Part model, mm, in its own coordinate system. Face numbers are marked on the shaded views. A direction names the side the tool comes from. Give positions to 0.01 mm unless a question says otherwise; leave off trailing zeros. Write each loop counter-clockwise with the first axis right and the second up, starting at its lowest first coordinate (ties: lowest second). Pieces come first, ordered by that corner, then holes. Notation, with made-up numbers: M 17,-27.75 L 24,-27.75 A24 cw 24,2.25 Z; hole C 51,-21.75 d9. An arc over 180 degrees is marked long. Answer as CSV lines item,"result". Start each with the question number.
Item 1: Band-saw the part on C-C, the plane x = -18.5. List the corners of the cut face in (y, z).
Item 2: 3-axis set-ups, long thin cutter, end or side, ignore diameter. For the marked faces 4 and 5: which of +Z, -Z, +X, -X, +Y, -Y reach the whole face in a straight line?
Item 3: Band-saw the part on A-A, the plane z = 10. List the corners of the cut face in (x, y), then the cut area to 3 significant figures.
Item 4: Band-saw the part on B-B, the plane x = -9. List the corners of the cut face in (y, z), then the cut area to 3 significant figures.
Item 5: Band-saw the part on D-D, the plane z = 4. List the corners of the cut face in (x, y), then the cut area to 3 significant figures.
Item 6: Wall check: L1, parallel to Z at x = -9, y = -3.4; L2, parallel to Y at x = -15, z = 10; L3, parallel to Y at x = -4.75, z = 12.5. Give the ranges that are in metal, low to high. Write a range as from..to.
Item 7: Pin check, flat tips, straight feed: pin 1 (1 mm diameter, centred on x = -13.5, z = 7, fed in from +Y); pin 2 (1.5 mm diameter, centred on y = 5.5, z = 18, fed in from +X); pin 3 (10 mm diameter, centred on x = -5.5, y = 23, fed in from -Z); pin 4 (4 mm diameter, centred on x = -11, y = 11, fed in from +Z). Stop position of each tip, or through.
Item 8: Two-plate mould, pull along Z, no slides. Class the marked faces 1, 2 and 3: +Z half, -Z half, draft (parallel to the pull), parting line (faces both ways), or undercut.
from build123d import *

# Parameters (mm, degrees)
SALIENTE_EXTRUIR1_DEPTH = 30
CROQUIS2_R              = 4.3
CORTAR_EXTRUIR1_DEPTH   = 21.5
CORTAR_EXTRUIR2_REACH   = 40
CROQUIS3_R              = 1.7


with BuildPart() as part:
    # Croquis1 → Saliente-Extruir1 (new body)
    with BuildSketch(Plane.XY):
        Polygon((0, 0), (-12.5, 0), (-12.5, 32), (-20.5, 32), (-20.5, -6), (0, -6), align=None)
    extrude(amount=SALIENTE_EXTRUIR1_DEPTH)

    # Croquis2 → Cortar-Extruir1 (cut, through all)
    with BuildSketch(Plane.ZY.offset(20.5)):
        with Locations((10, 22)):
            Circle(CROQUIS2_R)
        with BuildLine():
            Line((30, 0), (19.230769231, 25.846153846))
            ThreePointArc((19.230769231, 25.846153846), (8.038838649, 31.805806757), (0, 22))
            Line((0, 22), (0, 21))
            Line((0, 21), (-1, 21))
            Line((-1, 21), (-1, 33))
            Line((-1, 33), (31, 33))
            Line((31, 33), (31, 0))
            Line((31, 0), (30, 0))
        make_face()
    extrude(amount=-CORTAR_EXTRUIR1_DEPTH, mode=Mode.SUBTRACT)

    # Croquis3 → Cortar-Extruir2 (cut, up to next)
    with BuildSketch(Plane.XZ.offset(6), mode=Mode.PRIVATE) as cortar_extruir2_sk1:
        with Locations((-9, 23)):
            Circle(CROQUIS3_R)
    cortar_extruir2_tool1 = extrude(cortar_extruir2_sk1.sketch, amount=-CORTAR_EXTRUIR2_REACH, mode=Mode.PRIVATE) & part.part
    add(cortar_extruir2_tool1.solids().sort_by_distance((-9, -6, 23))[0], mode=Mode.SUBTRACT)
    # Croquis3 → Cortar-Extruir2 (cut, up to next)
    with BuildSketch(Plane.XZ.offset(6), mode=Mode.PRIVATE) as cortar_extruir2_sk2:
        with Locations((-9, 7)):
            Circle(CROQUIS3_R)
    cortar_extruir2_tool2 = extrude(cortar_extruir2_sk2.sketch, amount=-CORTAR_EXTRUIR2_REACH, mode=Mode.PRIVATE) & part.part
    add(cortar_extruir2_tool2.solids().sort_by_distance((-9, -6, 7))[0], mode=Mode.SUBTRACT)


solid = part.part
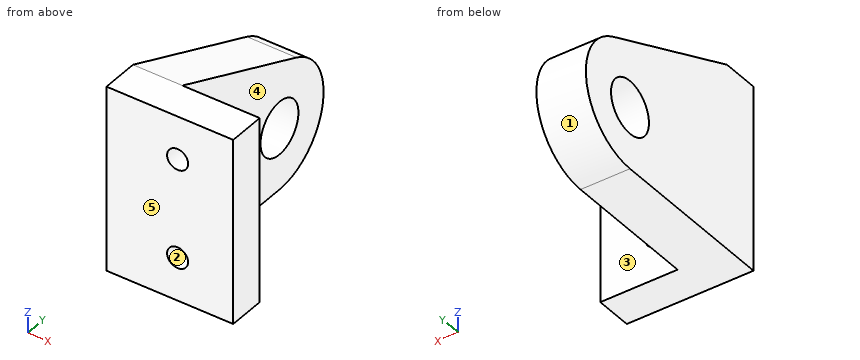
Output:
1,outline,"M -6,0 L 22,0 A10 ccw 25.85,19.23 L 0,30 L -6,30 Z; hole C 22,10 d8.6"
2,face 4,"+Z, -Z, +X, +Y"
2,face 5,"+Z, -Z, +X, -X, -Y"
3,outline,"M -20.5,-6 L 0,-6 L 0,0 L -12.5,0 L -12.5,17.7 L -20.5,17.7 Z; M -20.5,26.3 L -12.5,26.3 L -12.5,32 L -20.5,32 Z"
3,area,"310 mm²"
4,outline,"M -6,0 L 0,0 L 0,5.3 L -6,5.3 Z; M -6,8.7 L 0,8.7 L 0,21.3 L -6,21.3 Z; M -6,24.7 L 0,24.7 L 0,30 L -6,30 Z"
4,area,"139 mm²"
5,outline,"M -20.5,-6 L 0,-6 L 0,0 L -12.5,0 L -12.5,30 L -20.5,30 Z"
5,area,"363 mm²"
6,L1,"0..5.3, 8.7..21.3, 24.7..30"
6,L2,"-6..17.7, 26.3..32"
6,L3,"-6..0"
7,pin 1,"y = 31.68"
7,pin 2,"x = -12.5"
7,pin 3,"through"
7,pin 4,"z = 25.97"
8,face 1,"parting line"
8,face 2,"undercut"
8,face 3,"draft"
